Geometry check sheet. Reference: the model listing, model coordinates, mm. Face numbers are marked on the shaded views. A direction names the side the tool comes from. Give positions to 0.01 mm unless a question says otherwise; leave off trailing zeros. Order: outer loops, then holes, each group sorted by start corner. A loop starts at its lowest first (then second) coordinate and runs counter-clockwise, first axis right, second up.
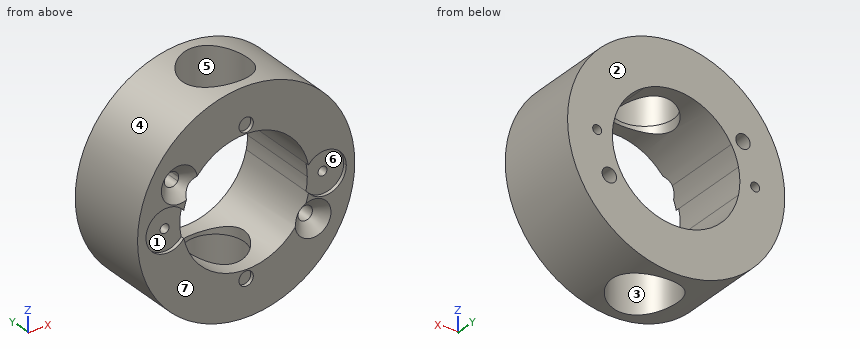
from build123d import *

# Parameters (mm, degrees)
F0_R          = 30.25
F0_R_2        = 2
F1_DEPTH      = 24
F0_R_3        = 1.25
F2_DEPTH      = 23
F5_R          = 9.125
F5_R_2        = 8
F6_DEPTH      = 25
F7_DEPTH      = 60
F7_DEPTH_BACK = 30
F8_START      = -37.5
F8_DEPTH      = 45.7


# Not quite as in the source:
# - a fillet or chamfer that OpenCascade refuses, or shapes differently, is made with other operations: its cross-section is extruded or revolved along the edge and cut away or added


with BuildPart() as f1:
    # F0 (on Front) → F1 (new body)
    with BuildSketch(Plane.XZ):
        Circle(F0_R)
        with Locations((0, -20.07)):
            Circle(F0_R_2, mode=Mode.SUBTRACT)
        with Locations((18.6195461814, -10.75)):
            Circle(F0_R_2, mode=Mode.SUBTRACT)
        with BuildLine():
            ThreePointArc((-16.6195461814, 10.75), (-16.6876945288, 10.2323619098), (-16.8874953738, 9.75))
            ThreePointArc((-16.8874953738, 9.75), (-20.5513978339, 11.2676380902), (-16.6195461814, 10.75))
        make_face(mode=Mode.SUBTRACT)
        with BuildLine():
            ThreePointArc((8.875, 15.3719509172), (14.3703479176, 10.4190019065), (17.369375, 3.6561334917))
            ThreePointArc((17.369375, 3.6561334917), (23.9351114309, 5.5736293158), (27.9, 0))
            ThreePointArc((27.9, 0), (23.9351114309, -5.5736293158), (17.369375, -3.6561334917))
            ThreePointArc((17.369375, -3.6561334917), (0, -17.75), (-17.369375, -3.6561334917))
            ThreePointArc((-17.369375, -3.6561334917), (-27.9, 0), (-17.369375, 3.6561334917))
            ThreePointArc((-17.369375, 3.6561334917), (-16.5773263107, 6.3446632999), (-15.3719509172, 8.875))
            ThreePointArc((-15.3719509172, 8.875), (-4.5940380506, 17.1451834166), (8.875, 15.3719509172))
        make_face(mode=Mode.SUBTRACT)
        with Locations((0, 20.07)):
            Circle(F0_R_2, mode=Mode.SUBTRACT)
    extrude(amount=F1_DEPTH)

    # F0 (on Front) → F2 (join)
    with BuildSketch(Plane.XZ):
        with BuildLine():
            ThreePointArc((-17.369375, 3.6561334917), (-27.9, 0), (-17.369375, -3.6561334917))
            ThreePointArc((-17.369375, -3.6561334917), (-17.75, 0), (-17.369375, 3.6561334917))
        make_face()
        with Locations((-22, 0)):
            Circle(F0_R_3, mode=Mode.SUBTRACT)
        with Locations((0, 20.07)):
            Circle(F0_R_2)
        with BuildLine():
            ThreePointArc((17.369375, 3.6561334917), (17.6545873111, 1.8379463744), (17.75, 0))
            ThreePointArc((17.75, 0), (17.6545873111, -1.8379463744), (17.369375, -3.6561334917))
            ThreePointArc((17.369375, -3.6561334917), (23.9351114309, -5.5736293158), (27.9, 0))
            ThreePointArc((27.9, 0), (23.9351114309, 5.5736293158), (17.369375, 3.6561334917))
        make_face()
        with Locations((22, 0)):
            Circle(F0_R_3, mode=Mode.SUBTRACT)
        with Locations((0, -20.07)):
            Circle(F0_R_2)
    extrude(amount=F2_DEPTH)

    # F3: chamfer of 3 on 2 edges, made by hand

    # F3_s1 → F3_t2 (revolve, cut)
    with BuildSketch(Plane.XY.offset(10.75)):
        Polygon((-13.6195461814, -24), (-16.6195461814, -21), (-16.6195461814, -24), align=None)
    revolve(axis=Axis((-18.6195461814, -24, 10.75), (0, -1, 0)), mode=Mode.SUBTRACT)

    # F3_s3 → F3_t4 (revolve, cut)
    with BuildSketch(Plane.XY.offset(-10.75)):
        Polygon((23.6195461814, -24), (20.6195461814, -21), (20.6195461814, -24), align=None)
    revolve(axis=Axis((18.6195461814, -24, -10.75), (0, -1, 0)), mode=Mode.SUBTRACT)

    # F5 (on offset) → F6 (cut)
    with BuildSketch(Plane.XY.offset(18.75)):
        with Locations((0, -12.125)):
            Circle(F5_R)
        with Locations((0, -12.125)):
            Circle(F5_R_2, mode=Mode.SUBTRACT)
    extrude(amount=F6_DEPTH, mode=Mode.SUBTRACT)

    # F5 (on offset) → F7 (cut, two sides)
    with BuildSketch(Plane.XY.offset(18.75)) as f7_sk:
        with Locations((0, -12.125)):
            Circle(F5_R_2)
    extrude(amount=-F7_DEPTH, mode=Mode.SUBTRACT)
    extrude(f7_sk.sketch, amount=F7_DEPTH_BACK, mode=Mode.SUBTRACT)

    # F5 (on offset) → F8 (cut)
    with BuildSketch(Plane.XY.offset(18.75).offset(F8_START)):
        with Locations((0, -12.125)):
            Circle(F5_R)
        with Locations((0, -12.125)):
            Circle(F5_R_2, mode=Mode.SUBTRACT)
    extrude(amount=-F8_DEPTH, mode=Mode.SUBTRACT)


solid = f1.part
Item 1: Gauge pin test, flat ends, axial feed: pin 1 (8 mm diameter, centred on x = 24, y = -3.5, fed in from +Z) (3 decimals); pin 2 (3 mm diameter, centred on y = -5, z = 4.5, fed in from -X); pin 3 (2 mm diameter, centred on x = -18.5, y = -10, fed in from +Z). Record the tip position at first contact, or that the pin passes through.
Reported:
pin 1: stops at z = 22.695
pin 2: stops at x = -30.1
pin 3: stops at z = 24.67
Item 2: Sectioned sample at D-D (y = -22). Enter the section's corners in (x, z) (3 decimals), and give its area (3 significant figures).
Reported:
outline: circle Ø60.5 at (0, 0); hole circle Ø2.5 at (-22, 0); hole circle Ø6 at (-18.62, 10.75); hole circle Ø35.5 at (0, 0); hole circle Ø6 at (18.62, -10.75); hole circle Ø2.5 at (22, 0)
area: 1,820 mm2
Item 3: Set-up check for the marked faces 1, 2 and 3: record each of +Z, -Z, +X, -X, +Y, -Y from which the full face is reachable in a straight line by a thin tool's end or side.
Reported:
face 1: -Y
face 2: +Z, -Z, +X, -X, +Y
face 3: -Z
Item 4: Draft check along X on the marked faces 4, 5, 6 and 7. Enter one of: released by +X, released by -X, zero draft, split by the parting line, or undercut.
Reported:
face 4: split by the parting line
face 5: undercut
face 6: undercut
face 7: zero draft
Item 5: Scan lines: L1, parallel to Z at x = 0, y = -23.3; L2, parallel to Z at x = -22, y = -20; L3, parallel to Z at x = -22, y = -23.3. Record each from-to range of solid material in increasing order.
Reported:
L1: z = -30.25 to -22.07, -18.07 to -17.75, 17.75 to 18.07, 22.07 to 30.25
L2: z = -20.76 to -1.25, 1.25 to 20.76
L3: z = -20.76 to -5.9, 5.9 to 8.09, 13.41 to 20.76
Item 6: Sectioned sample at A-A (y = -14). Give the number of separate pieces and of enclosed holes in the cut face, and give its area (3 significant figures).
Reported:
separate pieces: 2
enclosed holes: 4
area: 1,410 mm2
Item 7: Sectioned sample at C-C (x = 10.5). Enter the section's corners in (y, z).
Reported:
outline: (-24, -28.37) - (0, -28.37) - (0, -14.31) - (-24, -14.31) - close; (-24, 14.31) - (0, 14.31) - (0, 28.37) - (-24, 28.37) - close
